Design review of the part shown in the three views and the two pictorial views. Dimensions are in mm from the part's minimum x, y and z. Give positions to 0.01 mm unless a question says otherwise; leave off trailing zeros. Order: outer loops, then holes, each group sorted by start corner. A loop starts at its lowest first (then second) coordinate and runs counter-clockwise, first axis right, second up. Notation, with made-up numbers: M 83.5,84 L 115.5,84 A19 cw 115.5,104 Z; hole C -33.75,28 d10. An arc over 180 degrees is marked long. Answer as a JSON object with one key per item and string values.
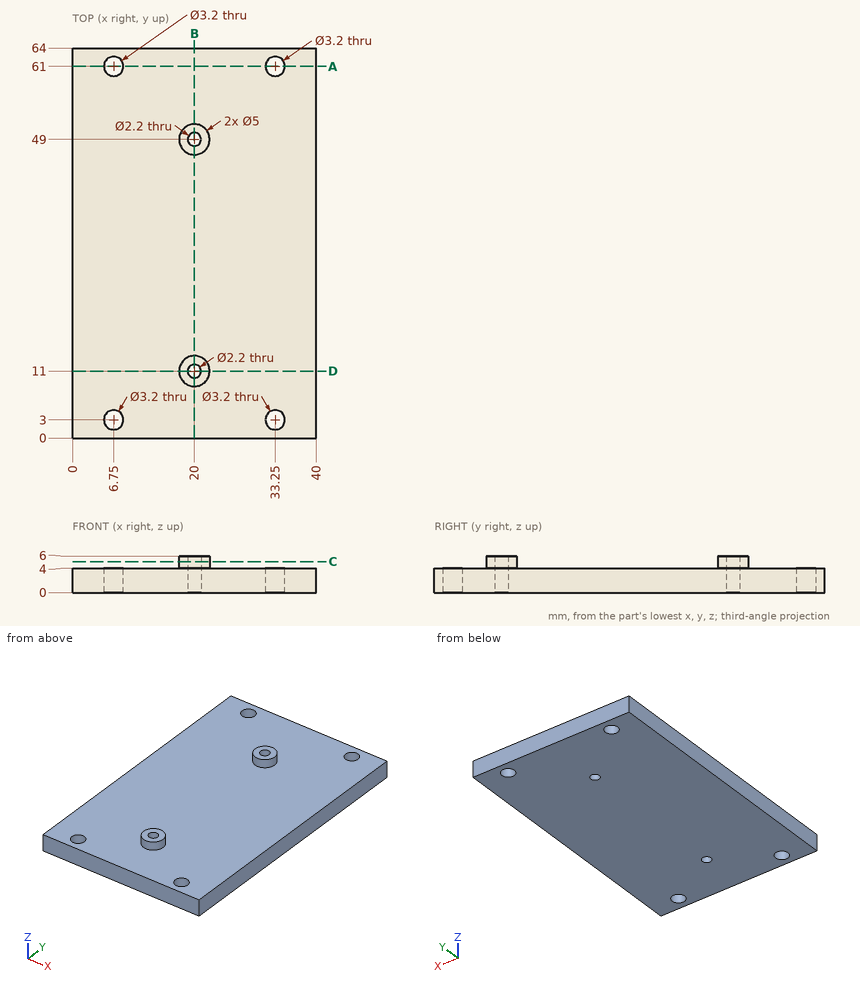
(1) To check wall thickness, follow L1, parallel to Y at x = 6.75, z = 2.25; L2, parallel to Y at x = 20, z = 4.3; L3, parallel to Y at x = 32.5, z = 3.1. State the ranges of each line that lie inside material, in increasing order. Write a range as from..to.
Checked values:
{"L1": "y = 0..1.4, 4.6..59.4, 62.6..64", "L2": "y = 8.5..9.9, 12.1..13.5, 46.5..47.9, 50.1..51.5", "L3": "y = 0..1.59, 4.41..59.59, 62.41..64"}
(2) We need section A-A (y = 61). Write out the cut boundary in (x, z), plus the area to 3 significant figures.
Checked values:
{"outline": "M 0,0 L 5.15,0 L 5.15,4 L 0,4 Z; M 8.35,0 L 31.65,0 L 31.65,4 L 8.35,4 Z; M 34.85,0 L 40,0 L 40,4 L 34.85,4 Z", "area": "134 mm^2"}
(3) We need section D-D (y = 11). Write out the cut boundary in (x, z).
Checked values:
{"outline": "M 0,0 L 18.9,0 L 18.9,6 L 17.5,6 L 17.5,4 L 0,4 Z; M 21.1,0 L 40,0 L 40,4 L 22.5,4 L 22.5,6 L 21.1,6 Z"}
(4) We need section B-B (x = 20). Write out the cut boundary in (y, z).
Checked values:
{"outline": "M 0,0 L 9.9,0 L 9.9,6 L 8.5,6 L 8.5,4 L 0,4 Z; M 12.1,0 L 47.9,0 L 47.9,6 L 46.5,6 L 46.5,4 L 13.5,4 L 13.5,6 L 12.1,6 Z; M 50.1,0 L 64,0 L 64,4 L 51.5,4 L 51.5,6 L 50.1,6 Z"}
(5) We need section C-C (z = 5.1). Write out the cut boundary in (x, y), plus the area to 3 significant figures.
Checked values:
{"outline": "C 20,11 d5; C 20,49 d5; hole C 20,11 d2.2; hole C 20,49 d2.2", "area": "31.7 mm^2"}
(6) Insertion check: pin 1 (6 mm diameter, centred on x = 7, y = 37.5, fed in from +Z). The pin has a flat end and moves straight along its axis. Give the tip position at first contact, or say it passes through.
Checked values:
{"pin 1": "stops at z = 4"}
